The drawing under review shows one solid part. Ordinate dimensions are in mm from its lowest x, y, z. A direction names the side the tool comes from. Coordinates: 2 decimals unless noted, no trailing zeros. Order: outer loops, then holes, each group sorted by start corner. A loop starts at its lowest first (then second) coordinate and runs counter-clockwise, first axis right, second up. Notation, with made-up numbers: (-33, 43.25) -> (18, 43.25) arc R12 cw to (18, 65.25) -> close; hole circle Ø7 at (87, -25.5). An arc over 180 degrees is marked (long way). Use a Markdown table: item, result. Add a question column.
Q1. Add section C-C (y = 99). State the section outline as (x, z) points.
Q2. Insertion check: pin 1 (3.5 mm diameter, centred on x = 6.75, y = 6.14, fed in from -Z); pin 2 (0.8 mm diameter, centred on y = 9.5, z = 47, fed in from +X); pin 3 (3 mm diameter, centred on x = 13, z = 38, fed in from -Y); pin 4 (1 mm diameter, centred on x = 62, z = 7.5, fed in from -Y) (1 decimal). Each pin has a flat end and moves straight along its axis. Give the tip position at first contact, or say it passes through.
Q3. Add section B-B (z = 29). State the section outline as (x, y) points (1 decimal), then the cut area to 3 significant figures.
Q4. Add section A-A (x = 6.75). State the section outline as (y, z) points (1 decimal), then the cut area to 3 significant figures.
Q5. Wall thickness on probe 1 along Y at (x, z) = (78, 11) (1 decimal): over which ranges is the line inside the solid? List them lowest first.
Q6. Machinability: for the marked faces 1 and 2, which of the approach directions +Z, -Z, +X, -X, +Y, -Y give a long, thin tool a straight path to every point of the face, cutting with its end or side? Answer none if there is none.
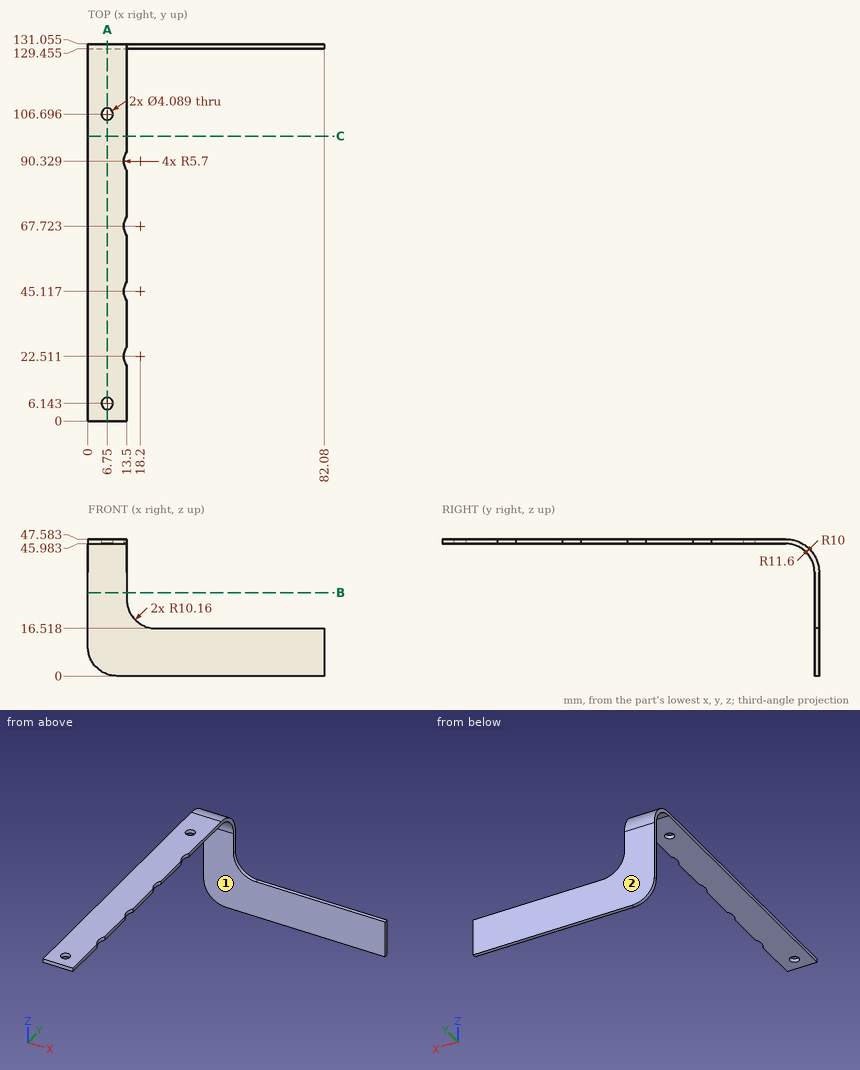
Established:
| question | item | result |
|---|---|---|
| 1 | outline | (0, 45.98) -> (13.5, 45.98) -> (13.5, 47.58) -> (0, 47.58) -> close |
| 2 | pin 1 | through |
| 2 | pin 2 | x = 13.5 |
| 2 | pin 3 | y = 128.82 |
| 2 | pin 4 | y = 129.5 |
| 3 | outline | (0, 129.5) -> (13.5, 129.5) -> (13.5, 131.1) -> (0, 131.1) -> close |
| 3 | area | 21.6 mm^2 |
| 4 | outline | (0, 46) -> (4.1, 46) -> (4.1, 47.6) -> (0, 47.6) -> close; (8.2, 46) -> (104.7, 46) -> (104.7, 47.6) -> (8.2, 47.6) -> close; (108.7, 46) -> (119.5, 46) arc R10 cw to (129.5, 36) -> (129.5, 0.6) -> (131.1, 0.6) -> (131.1, 36) arc R11.6 ccw to (119.5, 47.6) -> (108.7, 47.6) -> close |
| 4 | area | 262 mm^2 |
| 5 | probe 1 | 129.5 to 131.1 |
| 6 | face 1 | -Z, +X, -X, -Y |
| 6 | face 2 | +Z, -Z, +X, -X, +Y |
